```python
from build123d import *

# Parameters (mm, degrees)
F0_R            = 15.8688012495
F0_R_2          = 1.190625
F1_DEPTH        = 5.08
F3_DEPTH        = 5.08
F3_COPIES_COUNT = 32


# Not quite as in the source:
# - a pattern or mirror of a feature is missing from the dataset's text; its kind, count and spacing are read off the source's solid


with BuildPart() as f1:
    # F0 (on Top) → F1 (new body)
    with BuildSketch(Plane.XY):
        Circle(F0_R)
        with Locations((0, -7.9375)):
            Circle(F0_R_2, mode=Mode.SUBTRACT)
        Polygon((-4.5827177617, 0), (-2.2913588808, 3.96875), (2.2913588808, 3.96875), (4.5827177617, 0), (2.2913588808, -3.96875), (-2.2913588808, -3.96875), align=None, mode=Mode.SUBTRACT)
    extrude(amount=F1_DEPTH)

    # F2 (on face) → F3 (cut, through all)
    with BuildSketch(Plane(origin=(0, 0, 0), x_dir=(1, 0, 0), z_dir=(0, 0, -1))):
        with BuildLine():
            Line((0.2746540111, 13.8873319852), (1.0847660613, 15.8316813917))
            ThreePointArc((1.0847660613, 15.8316813917), (0, 15.8688012495), (-1.0847660613, 15.8316813917))
            Line((-1.0847660613, 15.8316813917), (-0.2746540111, 13.8873319852))
            ThreePointArc((-0.2746540111, 13.8873319852), (0, 13.7042263959), (0.2746540111, 13.8873319852))
        make_face()
    f3 = extrude(amount=-F3_DEPTH, mode=Mode.SUBTRACT)

    # F3_copies: F3 ×32 about axis
    f3_copies_axis = Axis((0, 0, 0), (0, 0, 1))
    for i in range(1, F3_COPIES_COUNT):
        add(f3.rotate(f3_copies_axis, i * 360 / F3_COPIES_COUNT), mode=Mode.SUBTRACT)


solid = f1.part
```
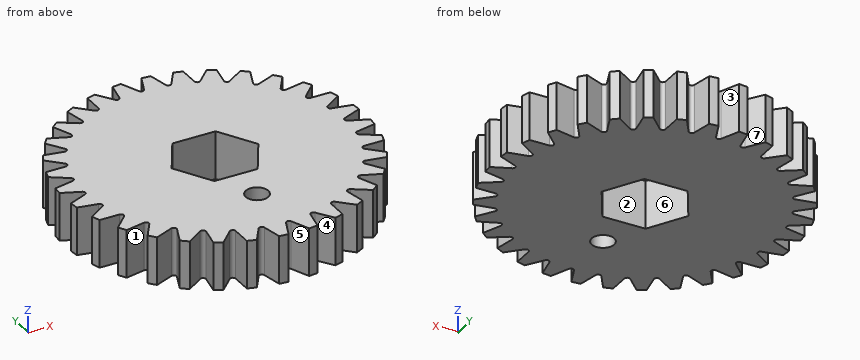
Geometry: final body of the model. Coordinates: model frame, mm. Face numbers are marked on the shaded views. A direction names the side the tool comes from. Round coordinates to 2 decimals unless told otherwise and drop trailing zeros. Write each loop counter-clockwise with the first axis right and the second up, starting at its lowest first coordinate (ties: lowest second). Pieces come first, ordered by that corner, then holes. Notation, with made-up numbers: (52.25, 15) -> (104.25, 15) arc R22 ccw to (104.25, 51) -> close; hole circle Ø5 at (85, -39.5). An arc over 180 degrees is marked (long way). Return JSON: item names as keys, results as strings.
Q1. Section B-B on z = 4.3. Give the number of separate pieces and of enclosed holes in the cut face, and give its area (3 significant figures).
From the geometry:
{"separate pieces": "1", "enclosed holes": "2", "area": "643 mm2"}
Q2. First-contact query: pin 1 Ø2 at (y, z) = (12, 1) entering from -X; pin 2 Ø2 at (y, z) = (0, 4) entering from +X; pin 3 Ø4 at (x, y) = (0, -7.94) entering from -Z. Flat tips, straight axial feed; report the tip coordinate or a pass-through.
From the geometry:
{"pin 1": "x = -10.43", "pin 2": "x = 15.63", "pin 3": "z = 0"}
Q3. Section A-A on x = 9. Return the cut outline in (y, z).
From the geometry:
{"outline": "(-12.1, 0) -> (12.1, 0) -> (12.1, 5.08) -> (-12.1, 5.08) -> close"}
Q4. Section C-C on x = -8.5. Return the cut outline in (y, z).
From the geometry:
{"outline": "(-11.76, 0) -> (11.76, 0) -> (11.76, 5.08) -> (-11.76, 5.08) -> close"}
Q5. Mould query, pull axis Y, two halves, no side actions, for the marked faces 1, 2, 3 and 4. Classes: +Y half, -Y half, draft (parallel to the pull), parting line (faces both ways), or undercut.
From the geometry:
{"face 1": "undercut", "face 2": "undercut", "face 3": "+Y half", "face 4": "-Y half"}
Q6. Set-up query: the marked faces 5, 6 and 7. Return all of +Z, -Z, +X, -X, +Y, -Y with unobstructed straight access to the full face (end or side cutting, diameter ignored); none if empty.
From the geometry:
{"face 5": "+Z, -Z, -Y", "face 6": "+Z, -Z", "face 7": "+Z, -Z, +Y"}
Q7. Ray query, line 1 (Y direction, x = 0, z = 2.7); line 2 (X direction, y = -14, z = 2.1); line 3 (X direction, y = 12.5, z = 3.6). Return the intervals inside material, ascending.
From the geometry:
{"line 1": "-13.7 to -9.13, -6.75 to -3.97, 3.97 to 13.7", "line 2": "-7.47 to -6.85, -5.06 to -3.27, -2.37 to -0.32, 0.32 to 2.37, 3.27 to 5.06, 6.85 to 7.47", "line 3": "-9.78 to -9.61, -7.64 to 7.64, 9.61 to 9.78"}
